Source: CAD feature listing. Evaluate the final solid. Frame: model axes, mm. A direction names the side the tool comes from. Give positions to 0.01 mm unless a question says otherwise; leave off trailing zeros. Write each loop counter-clockwise with the first axis right and the second up, starting at its lowest first coordinate (ties: lowest second). Pieces come first, ordered by that corner, then holes. Notation, with made-up numbers: (55, 54.5) - (92, 54.5) arc R15 ccw to (92, 74.5) - close; hole circle Ø2 at (56, -3.5). An arc over 180 degrees is marked (long way). One line per question, with ' | ' between items. Start each with the question number.
(1) Access query for faces 1 (the flat face through (-4, 31, 30)), 2 (the flat face through (0, -1, 2)), 3 (the flat face through (-2, 21.15, 26)). Directions: +Z, -Z, +X, -X, +Y, -Y. A direction counts if a zero-diameter tool reaches every point of the face in a straight line with its end or side. Return the directions, or none.
(2) Draft query along Z for faces 4 (the cylindrical face through (-29.88, -6.69, 3.45)), 5 (the flat face through (-17, 11, 0)), 6 (the cylindrical face through (-1.97, 28.67, 25.48)), 7 (the flat face through (-2, 33, 45)). Return one class per face: +Z half, -Z half, draft (parallel to the pull), parting line (faces both ways), or undercut.
(3) Ray query, line 1 (Y direction, x = -6.15, z = 4.5); line 2 (Y direction, x = -13, z = 11); line 3 (Y direction, x = -21.15, z = 4). Return the intervals inside material, ascending. Write a range as [from, to].
(4) Section D-D, the plane z = 23. Return loops of the section in (x, y), plus the area to 3 significant figures.
(5) Section C-C, the plane x = -36.15. Return loops of the section in (y, z), plus the area to 3 significant figures.
(6) Section A-A, the plane z = 17.5. Return loops of the section in (x, y), plus the area to 3 significant figures.
(7) Pin query (flat end, axial travel): pin 1 (1.5 mm diameter, centred on x = -14, z = 20, fed in from +Y); pin 2 (6 mm diameter, centred on y = 29, z = 23, fed in from -X); pin 3 (21 mm diameter, centred on x = -21.5, y = 7.5, fed in from +Z). Return the tip coordinate at first contact, or that it passes through.
(8) Section B-B, the plane y = 0. Return loops of the section in (x, z), plus the area to 3 significant figures.
```python
from build123d import *

# Parameters (mm, degrees)
SKETCH001_W  = 24.85
SKETCH001_H  = 38
SKETCH001_R  = 2.5
PAD001_DEPTH = 4
PAD002_DEPTH = 9
SKETCH_W     = 42.3
SKETCH_H     = 92
SKETCH_R     = 1.75
SKETCH_R_2   = 11
PAD_DEPTH    = 7
PAD003_DEPTH = 9


with BuildPart() as support:
    # Sketch001 → Pad001 (new body)
    with BuildSketch(Plane.YZ):
        with Locations((-33.575, 26)):
            Rectangle(SKETCH001_W, SKETCH001_H)
        with Locations((-29, 23)):
            Circle(SKETCH001_R, mode=Mode.SUBTRACT)
        with Locations((33.575, 26)):
            Rectangle(SKETCH001_W, SKETCH001_H)
        with Locations((29, 23)):
            Circle(SKETCH001_R, mode=Mode.SUBTRACT)
    extrude(amount=-PAD001_DEPTH)


with BuildPart() as pad002:
    # Sketch002 → Pad002 (new body)
    with BuildSketch(Plane.XZ.offset(46)):
        Polygon((-4, 27), (-4, 7), (-24, 7), align=None)
    extrude(amount=-PAD002_DEPTH)


with BuildPart() as obj1:
    # Sketch → Pad (new body)
    with BuildSketch(Plane.XY):
        with Locations((-21.15, 0)):
            Rectangle(SKETCH_W, SKETCH_H)
        with Locations((-6.15, 15)):
            Circle(SKETCH_R, mode=Mode.SUBTRACT)
        with Locations((-21.15, 0)):
            Circle(SKETCH_R_2, mode=Mode.SUBTRACT)
        with Locations((-36.15, 15)):
            Circle(SKETCH_R, mode=Mode.SUBTRACT)
        with Locations((-36.15, -15)):
            Circle(SKETCH_R, mode=Mode.SUBTRACT)
        with Locations((-6.15, -15)):
            Circle(SKETCH_R, mode=Mode.SUBTRACT)
    extrude(amount=PAD_DEPTH)


with BuildPart() as fixation:
    # Sketch003 → Pad003 (new body)
    with BuildSketch(Plane.XZ.offset(-46)):
        Polygon((-4, 27), (-4, 7), (-24, 7), align=None)
    extrude(amount=PAD003_DEPTH)

    # Fusion: union support, Pad002, obj1
    add(support.part)
    add(pad002.part)
    add(obj1.part)


solid = fixation.part
```
Check sheet entries:
1) face 1: +Z, -X | face 2: +Z, -Z, +X, +Y, -Y | face 3: +Z, +X, -X
2) face 4: draft | face 5: -Z half | face 6: undercut | face 7: +Z half
3) line 1: [-46, -16.75], [-13.25, 13.25], [16.75, 46] | line 2: [-46, -37], [37, 46] | line 3: [-46, -11], [11, 46]
4) outline: (-8, -46) - (0, -46) - (0, -31.5) - (-4, -31.5) - (-4, -37) - (-8, -37) - close; (-8, 37) - (-4, 37) - (-4, 31.5) - (0, 31.5) - (0, 46) - (-8, 46) - close; (-4, -26.5) - (0, -26.5) - (0, -21.15) - (-4, -21.15) - close; (-4, 21.15) - (0, 21.15) - (0, 26.5) - (-4, 26.5) - close | area: 231 mm²
5) outline: (-46, 0) - (-16.75, 0) - (-16.75, 7) - (-46, 7) - close; (-13.25, 0) - (13.25, 0) - (13.25, 7) - (-13.25, 7) - close; (16.75, 0) - (46, 0) - (46, 7) - (16.75, 7) - close | area: 595 mm²
6) outline: (-13.5, -46) - (0, -46) - (0, -21.15) - (-4, -21.15) - (-4, -37) - (-13.5, -37) - close; (-13.5, 37) - (-4, 37) - (-4, 21.15) - (0, 21.15) - (0, 46) - (-13.5, 46) - close | area: 370 mm²
7) pin 1: through | pin 2: x = -4 | pin 3: z = 7
8) outline: (-42.3, 0) - (-32.15, 0) - (-32.15, 7) - (-42.3, 7) - close; (-10.15, 0) - (0, 0) - (0, 7) - (-10.15, 7) - close | area: 142 mm²
